Job drawing, mm, ordinate dimensions from the low corner. One solid piece. A direction names the side the tool comes from. Give positions to 0.01 mm unless a question says otherwise; leave off trailing zeros. Write each loop counter-clockwise with the first axis right and the second up, starting at its lowest first coordinate (ties: lowest second). Pieces come first, ordered by that corner, then holes. Notation, with made-up numbers: (4, 72) - (19, 72) arc R25 cw to (19, 107) - close; hole circle Ø5 at (45, 35.5). An arc over 180 degrees is marked (long way). Put each result on its own line as item: value. Start each with the question number.
1. Cut at A-A on z = 35.5. List the corners of the cut face in (x, y), and give its area (3 significant figures).
2. Tool access for the marked faces 1 and 2: list every direction of +Z, -Z, +X, -X, +Y, -Y with a clear straight run to the whole face (end or side of a thin tool).
3. Drop flat-ended pins along their axis: pin 1 (5 mm diameter, centred on x = 25, y = 6, fed in from +Z); pin 2 (3 mm diameter, centred on y = 8, z = 17, fed in from -X); pin 3 (1 mm diameter, centred on x = 58, y = 4.5, fed in from -Z); pin 4 (10 mm diameter, centred on x = 47, z = 19.5, fed in from -Y). Give the stop position or say it passes through.
4. Cut at C-C on y = 3.75. List the corners of the cut face in (x, z), and give its area (3 significant figures).
5. Cut at D-D on x = 28. List the corners of the cut face in (y, z).
6. Cut at B-B on x = 8. List the corners of the cut face in (y, z), and give its area (3 significant figures).
7. Wall check: line 1 (X direction, y = 5, z = 29.5); line 2 (Z direction, x = 24.5, y = 4.25); line 3 (Z direction, x = 29, y = 2.5). Give the ranges that are in metal, low to high.
8. Mould opens along Z. For the marked faces 3, 4, 5 and 6 say: +Z half, -Z half, draft (parallel to the pull), parting line (faces both ways), or undercut.
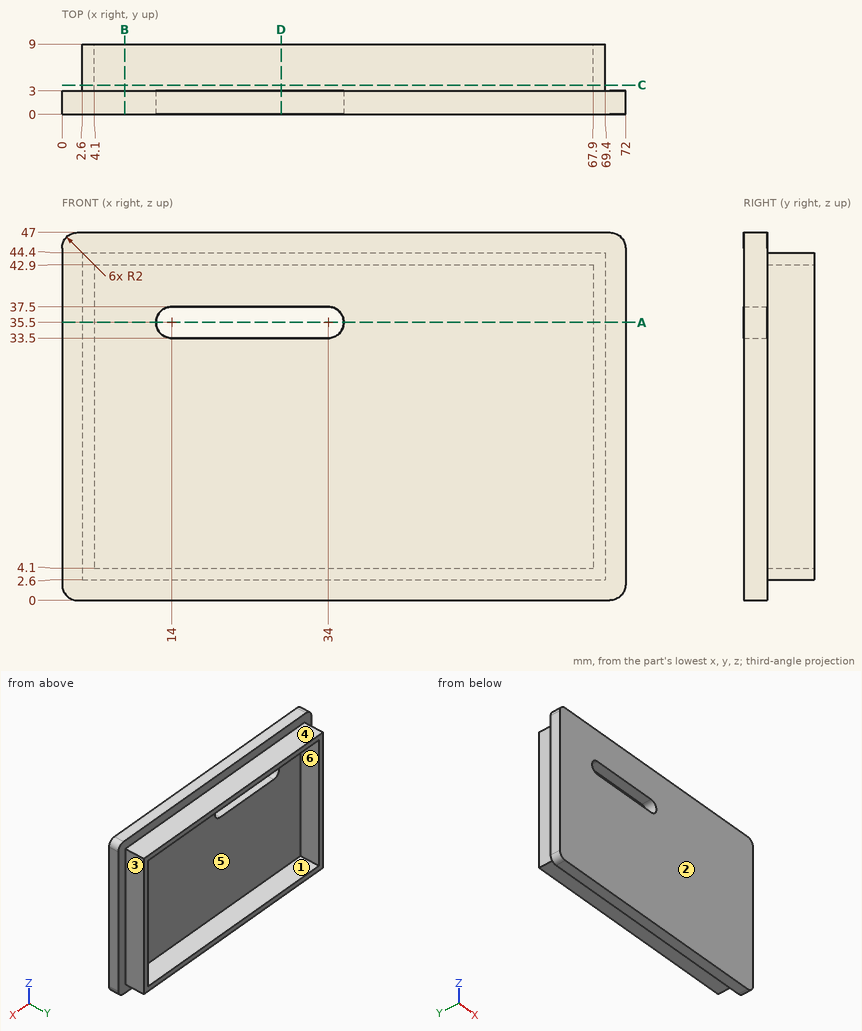
Report:
1. outline: (0, 0) - (12, 0) - (12, 3) - (4.1, 3) - (4.1, 9) - (2.6, 9) - (2.6, 3) - (0, 3) - close; (36, 0) - (72, 0) - (72, 3) - (69.4, 3) - (69.4, 9) - (67.9, 9) - (67.9, 3) - (36, 3) - close
1. area: 162 mm²
2. face 1: +Y
2. face 2: +Z, -Z, +X, -X, -Y
3. pin 1: stops at z = 44.4
3. pin 2: stops at x = 2.6
3. pin 3: stops at z = 2.6
3. pin 4: stops at y = 0
4. outline: (2.6, 2.6) - (69.4, 2.6) - (69.4, 44.4) - (2.6, 44.4) - close; hole (4.1, 4.1) - (67.9, 4.1) - (67.9, 42.9) - (4.1, 42.9) - close
4. area: 317 mm²
5. outline: (0, 0) - (3, 0) - (3, 2.6) - (9, 2.6) - (9, 4.1) - (3, 4.1) - (3, 33.5) - (0, 33.5) - close; (0, 37.5) - (3, 37.5) - (3, 42.9) - (9, 42.9) - (9, 44.4) - (3, 44.4) - (3, 47) - (0, 47) - close
6. outline: (0, 0) - (3, 0) - (3, 2.6) - (9, 2.6) - (9, 4.1) - (3, 4.1) - (3, 42.9) - (9, 42.9) - (9, 44.4) - (3, 44.4) - (3, 47) - (0, 47) - close
6. area: 159 mm²
7. line 1: x = 2.6 to 4.1, 67.9 to 69.4
7. line 2: z = 2.6 to 4.1, 42.9 to 44.4
7. line 3: z = 0 to 33.5, 37.5 to 47
8. face 3: draft
8. face 4: +Z half
8. face 5: undercut
8. face 6: undercut
